CAD build for the part. Positions are in the model's coordinates, mm. Give positions to 0.01 mm unless a question says otherwise; leave off trailing zeros. Order: outer loops, then holes, each group sorted by start corner. A loop starts at its lowest first (then second) coordinate and runs counter-clockwise, first axis right, second up.
Item 1: Two-plate mould, pull along X, no slides. Class faces 1 (the flat face through (2, 4, 2)), 2 (the cylindrical face through (-64.154, 2.028, 65.749)): released by +X, released by -X, zero draft, split by the parting line, or undercut.
Item 2: Flat gauge pins, fed straight in: P1, Ø2, axis at y = 2, z = -37.5, coming from the +X side; P2, Ø2, axis at y = 1, z = -127.5, coming from the -X side; P3, Ø2, axis at x = 126.5, y = 1.5, coming from the -Z side. Where does each tip first touch, or does it go through?
Item 3: Band-saw the part on D-D on z = -81.5. Give the cut face in (x, y), plus the area to 3 significant figures.
Item 4: Wall check: L1, parallel to X at y = 2.6, z = 62.2; L2, parallel to X at y = 1.7, z = -2.3; L3, parallel to X at y = 2.2, z = -76. Give the ranges that are in metal, low to high.
Item 5: Band-saw the part on B-B on x = -66. Give the cut face in (y, z).
Item 6: Band-saw the part on C-C on x = 66. Give the cut face in (y, z), plus the area to 3 significant figures.
Item 7: Band-saw the part on A-A on z = 62.2. Give the cut face in (x, y).
Autodesk Inventor part; units mm, degrees
ref_plane "YZ Plane" through (0, 0, 0) normal (1, 0, 0) x (0, 1, 0)
ref_plane "XZ Plane" through (0, 0, 0) normal (0, 1, 0) x (-1, 0, 0)
ref_plane "XY Plane" through (0, 0, 0) normal (0, 0, 1) x (1, 0, 0)
sketch "Sketch1" plane through (0, 0, 0) normal (0, 1, 0) x (-1, 0, 0)
  line L0 (-125, 125) -> (125, 125)
  line L1 (125, 125) -> (125, -125)
  line L2 (125, -125) -> (-125, -125)
  line L3 (-125, -125) -> (-125, 125)
  line L4 (-125, 125) -> (125, -125) construction
  line L5 (125, 125) -> (-125, -125) construction
  line L6 (125, -125) -> (75, -125)
  line L7 (75, -125) -> (75, -129)
  line L8 (75, -129) -> (125, -129)
  line L9 (125, -129) -> (125, -125)
  line L10 (125, -125) -> (129, -125)
  line L11 (129, -125) -> (129, -75)
  line L12 (129, -75) -> (125, -75)
  line L13 (125, -75) -> (125, -125)
  line L14 (-125, -125) -> (-129, -125)
  line L15 (-129, -125) -> (-129, -75)
  line L16 (-129, -75) -> (-125, -75)
  line L17 (-125, -75) -> (-125, -125)
  line L18 (125, 125) -> (75, 125)
  line L19 (75, 125) -> (75, 129)
  line L20 (75, 129) -> (125, 129)
  line L21 (125, 129) -> (125, 125)
  line L22 (75, -129) -> (75, -125)
  line L23 (75, -125) -> (25, -125)
  line L24 (25, -125) -> (25, -129)
  line L25 (25, -129) -> (75, -129)
  line L26 (25, -129) -> (25, -125)
  line L27 (25, -125) -> (-25, -125)
  line L28 (-25, -125) -> (-25, -129)
  line L29 (-25, -129) -> (25, -129)
  line L30 (-25, -129) -> (-25, -125)
  line L31 (-25, -125) -> (-75, -125)
  line L32 (-75, -125) -> (-75, -129)
  line L33 (-75, -129) -> (-25, -129)
  line L34 (-75, -129) -> (-75, -125)
  line L35 (-75, -125) -> (-125, -125)
  line L36 (-125, -125) -> (-125, -129)
  line L37 (-125, -129) -> (-75, -129)
  line L38 (125, -75) -> (129, -75)
  line L39 (125, -25) -> (125, -75)
  line L40 (129, -25) -> (125, -25)
  line L41 (129, -75) -> (129, -25)
  line L42 (125, -25) -> (129, -25)
  line L43 (125, 25) -> (125, -25)
  line L44 (129, 25) -> (125, 25)
  line L45 (129, -25) -> (129, 25)
  line L46 (125, 25) -> (129, 25)
  line L47 (125, 75) -> (125, 25)
  line L48 (129, 75) -> (125, 75)
  line L49 (129, 25) -> (129, 75)
  line L50 (125, 75) -> (129, 75)
  line L51 (125, 125) -> (125, 75)
  line L52 (129, 125) -> (125, 125)
  line L53 (129, 75) -> (129, 125)
  line L54 (-125, -75) -> (-129, -75)
  line L55 (-129, -75) -> (-129, -25)
  line L56 (-129, -25) -> (-125, -25)
  line L57 (-125, -25) -> (-125, -75)
  line L58 (-125, -25) -> (-129, -25)
  line L59 (-129, -25) -> (-129, 25)
  line L60 (-129, 25) -> (-125, 25)
  line L61 (-125, 25) -> (-125, -25)
  line L62 (-125, 25) -> (-129, 25)
  line L63 (-129, 25) -> (-129, 75)
  line L64 (-129, 75) -> (-125, 75)
  line L65 (-125, 75) -> (-125, 25)
  line L66 (-125, 75) -> (-129, 75)
  line L67 (-129, 75) -> (-129, 125)
  line L68 (-129, 125) -> (-125, 125)
  line L69 (-125, 125) -> (-125, 75)
  line L70 (75, 125) -> (25, 125)
  line L71 (25, 125) -> (25, 129)
  line L72 (25, 129) -> (75, 129)
  line L73 (75, 129) -> (75, 125)
  line L74 (25, 125) -> (-25, 125)
  line L75 (-25, 125) -> (-25, 129)
  line L76 (-25, 129) -> (25, 129)
  line L77 (25, 129) -> (25, 125)
  line L78 (-25, 125) -> (-75, 125)
  line L79 (-75, 125) -> (-75, 129)
  line L80 (-75, 129) -> (-25, 129)
  line L81 (-25, 129) -> (-25, 125)
  line L82 (-75, 125) -> (-125, 125)
  line L83 (-125, 125) -> (-125, 129)
  line L84 (-125, 129) -> (-75, 129)
  line L85 (-75, 129) -> (-75, 125)
  point P0 (0, 0)
  dimension "d0" = 250
  dimension "d1" = 250
  dimension "d2" = 50
  dimension "d3" = 4
  dimension "d4" = 4
  dimension "d5" = 50
  dimension "d6" = 4
  dimension "d7" = 50
  dimension "d8" = 50
  dimension "d9" = 4
  dimension "d12" = 50
  dimension "d19" = 50
  dimension "d26" = 50
  dimension "d33" = 50
extrude "Extrusion1" add sketch "Sketch1" along normal blind 4 contours L83 L84 L79 L0 | L0 L1 L2 L3 | L3 L64 L67 L68 | L75 L76 L71 L0 | L3 L56 L59 L60 | L19 L20 L21 L0 | L3 L14 L15 L16 | L52 L53 L48 L1 | L2 L32 L37 L36 | L44 L45 L40 L1 | L2 L24 L29 L28 | L12 L11 L10 L1 | L2 L9 L8 L7
sketch "Sketch2" plane through (0, 4, 0) normal (0, 1, 0) x (1, 0, 0)
  line L0 (25, -125) -> (75, -125) construction
  circle A0 centre (0, 2.3) radius 3.5
  line L1 (-8.45, 2.3) -> (8.45, 2.3) construction
  line L2 (-8.45, 1.0705) -> (8.45, 1.0705) construction
  line L3 (8.45, 3.5295) -> (-8.45, 3.5295) construction
  arc A1 (-8.45, 3.5295) -> (-8.45, 1.0705) centre (-8.45, 2.3) ccw construction
  arc A2 (8.45, 1.0705) -> (8.45, 3.5295) centre (8.45, 2.3) ccw construction
  circle A3 centre (8.45, 2.3) radius 1.2295
  circle A4 centre (-8.45, 2.3) radius 1.2295
  circle A5 centre (-66, -62.2) radius 4
  circle A6 centre (66, -62.2) radius 4
  line L4 (0, 180.6) -> (0, -180.6) construction
  line L5 (-93.2324, -124) -> (95.467, -124) construction
  line L6 (-129, -125) -> (-125, -125)
  line L7 (25, -29.4721) -> (29.2426, -25.2294)
  line L8 (44.799, -9.6731) -> (47.6274, -12.5015)
  line L9 (47.6274, -12.5015) -> (43.3848, -16.7442)
  line L10 (27.8284, -32.3005) -> (25, -29.4721)
  line L11 (34.8995, -39.3716) -> (39.1421, -35.1289)
  line L12 (54.6985, -19.5726) -> (57.5269, -22.401)
  line L13 (57.5269, -22.401) -> (53.2843, -26.6437)
  line L14 (37.7279, -42.2) -> (34.8995, -39.3716)
  line L15 (40.5563, -13.9157) -> (43.3848, -16.7442)
  line L16 (29.2426, -25.2294) -> (32.0711, -28.0579)
  line L17 (39.1421, -35.1289) -> (41.9706, -37.9574)
  line L18 (50.4558, -23.8152) -> (53.2843, -26.6437)
  line L19 (40.5563, -13.9157) -> (44.799, -9.6731)
  line L20 (29.2426, -25.2294) -> (40.5563, -13.9157) construction
  line L21 (43.3848, -16.7442) -> (32.0711, -28.0579) construction
  line L22 (50.4558, -23.8152) -> (54.6985, -19.5726)
  line L23 (53.2843, -26.6437) -> (41.9706, -37.9574) construction
  line L24 (32.0711, -28.0579) -> (27.8284, -32.3005)
  line L25 (39.1421, -35.1289) -> (50.4558, -23.8152) construction
  line L26 (41.9706, -37.9574) -> (37.7279, -42.2)
  point P0 (0, 0)
  point P1 (26.4142, -30.8863)
  dimension "d46" = 7
  dimension "d47" = 16.9
  dimension "d48" = 1.2295
  dimension "d52" = 8
  dimension "d53" = 132
  dimension "d54" = 61.8
  dimension "d55" = 1
  dimension "d56" = 64.5
  dimension "d57" = 10
  dimension "d58" = 4
  dimension "d59" = 6
  dimension "d60" = 6
  dimension "d61" = 45
  dimension "d62" = 20
  dimension "d63" = 28
  dimension "d64" = 25
extrude "Extrusion2" cut sketch "Sketch2" against normal up to next
sketch "Sketch3" plane through (0, 4, 0) normal (0, 1, 0) x (1, 0, 0)
  point P0 (0, 0)
sketch "Sketch4" plane through (0, 4, 0) normal (0, 1, 0) x (1, 0, 0)
  circle A0 centre (75, 75) radius 15
  line L0 (125, 25) -> (125, 75)
  line L1 (75, 125) -> (25, 125)
  point P0 (0, 0)
  dimension "d65" = 30
  dimension "d66" = 50
  dimension "d67" = 50
extrude "Extrusion3" cut sketch "Sketch4" against normal through all
sketch "Sketch5" plane through (0, 4, 0) normal (0, 1, 0) x (1, 0, 0)
  circle A0 centre (75, 75) radius 15
  line L0 (54.6985, -19.5726) -> (57.5269, -22.401)
  line L1 (57.5269, -22.401) -> (53.2843, -26.6437)
  line L2 (53.2843, -26.6437) -> (50.4558, -23.8152)
  line L3 (50.4558, -23.8152) -> (54.6985, -19.5726)
  circle A1 centre (8.45, 2.3) radius 1.2295
  circle A2 centre (0, 2.3) radius 3.5
  line L4 (39.1421, -35.1289) -> (41.9706, -37.9574)
  line L5 (41.9706, -37.9574) -> (37.7279, -42.2)
  line L6 (37.7279, -42.2) -> (34.8995, -39.3716)
  line L7 (34.8995, -39.3716) -> (39.1421, -35.1289)
  line L8 (44.799, -9.6731) -> (47.6274, -12.5015)
  line L9 (47.6274, -12.5015) -> (43.3848, -16.7442)
  line L10 (43.3848, -16.7442) -> (40.5563, -13.9157)
  line L11 (40.5563, -13.9157) -> (44.799, -9.6731)
  circle A3 centre (66, -62.2) radius 4
  circle A4 centre (-8.45, 2.3) radius 1.2295
  circle A5 centre (-66, -62.2) radius 4
  line L12 (29.2426, -25.2294) -> (32.0711, -28.0579)
  line L13 (32.0711, -28.0579) -> (27.8284, -32.3005)
  line L14 (27.8284, -32.3005) -> (25, -29.4721)
  line L15 (25, -29.4721) -> (29.2426, -25.2294)
  line L16 (-129, -125) -> (-125, -125)
  line L17 (-125, -125) -> (-125, -129)
  line L18 (-125, -129) -> (-75, -129)
  line L19 (-75, -129) -> (-75, -125)
  line L20 (-75, -125) -> (-25, -125)
  line L21 (-25, -125) -> (-25, -129)
  line L22 (-25, -129) -> (25, -129)
  line L23 (25, -129) -> (25, -125)
  line L24 (25, -125) -> (75, -125)
  line L25 (75, -125) -> (75, -129)
  line L26 (75, -129) -> (125, -129)
  line L27 (125, -129) -> (125, -125)
  line L28 (125, -125) -> (129, -125)
  line L29 (129, -125) -> (129, -75)
  line L30 (129, -75) -> (125, -75)
  line L31 (125, -75) -> (125, -25)
  line L32 (125, -25) -> (129, -25)
  line L33 (129, -25) -> (129, 25)
  line L34 (129, 25) -> (125, 25)
  line L35 (125, 25) -> (125, 75)
  line L36 (125, 75) -> (129, 75)
  line L37 (129, 75) -> (129, 125)
  line L38 (129, 125) -> (125, 125)
  line L39 (125, 125) -> (125, 129)
  line L40 (125, 129) -> (75, 129)
  line L41 (75, 129) -> (75, 125)
  line L42 (75, 125) -> (25, 125)
  line L43 (25, 125) -> (25, 129)
  line L44 (25, 129) -> (-25, 129)
  line L45 (-25, 129) -> (-25, 125)
  line L46 (-25, 125) -> (-75, 125)
  line L47 (-75, 125) -> (-75, 129)
  line L48 (-75, 129) -> (-125, 129)
  line L49 (-125, 129) -> (-125, 125)
  line L50 (-125, 125) -> (-129, 125)
  line L51 (-129, 125) -> (-129, 75)
  line L52 (-129, 75) -> (-125, 75)
  line L53 (-125, 75) -> (-125, 25)
  line L54 (-125, 25) -> (-129, 25)
  line L55 (-129, 25) -> (-129, -25)
  line L56 (-129, -25) -> (-125, -25)
  line L57 (-125, -25) -> (-125, -75)
  line L58 (-125, -75) -> (-129, -75)
  line L59 (-129, -75) -> (-129, -125)
  line L60 (-80.4142, -24.3431) -> (-77.5858, -21.5147)
  line L61 (-77.5858, -21.5147) -> (-81.8284, -17.2721)
  line L62 (-81.8284, -17.2721) -> (-84.6569, -20.1005)
  line L63 (-84.6569, -20.1005) -> (-80.4142, -24.3431)
  line L64 (-79, -30) -> (-71.9289, -22.9289) construction
  line L65 (-83.2426, -18.6863) -> (-79, -22.9289) construction
  line L66 (-79, -22.9289) -> (-75.4645, -26.4645) construction
  point P0 (0, 0)
  dimension "d70" = 45
  dimension "d71" = 4
  dimension "d72" = 6
  dimension "d73" = 10
  dimension "d74" = 95
  dimension "d75" = 46
  dimension "d78" = 5
extrude "Extrusion4" cut sketch "Sketch5" against normal through all contours L63 L62 L61 L60
properties part number "FloorPlateBottom_V2" material "Wood (Oak)"
The answers:
1. face 1: zero draft
1. face 2: undercut
2. P1: stops at x = 125
2. P2: stops at x = -125
2. P3: stops at z = -125
3. outline: (-129, 0) - (61.48, 0) - (61.48, 4) - (-129, 4) - close; (88.52, 0) - (129, 0) - (129, 4) - (88.52, 4) - close
3. area: 924 mm2
4. L1: x = -125 to -70, -62 to 62, 70 to 125
4. L2: x = -129 to -9.68, -7.22 to -3.5, 3.5 to 7.22, 9.68 to 129
4. L3: x = -129 to 60.03, 89.97 to 129
5. outline: (0, -125) - (4, -125) - (4, 58.2) - (0, 58.2) - close; (0, 66.2) - (4, 66.2) - (4, 125) - (0, 125) - close
6. outline: (0, -125) - (4, -125) - (4, -87) - (0, -87) - close; (0, -63) - (4, -63) - (4, 58.2) - (0, 58.2) - close; (0, 66.2) - (4, 66.2) - (4, 125) - (0, 125) - close
6. area: 872 mm2
7. outline: (-125, 0) - (-70, 0) - (-70, 4) - (-125, 4) - close; (-62, 0) - (62, 0) - (62, 4) - (-62, 4) - close; (70, 0) - (125, 0) - (125, 4) - (70, 4) - close
